Geometry: final body of the model. Coordinates: model frame, mm. A direction names the side the tool comes from. Coordinates: 2 decimals unless noted, no trailing zeros. Order: outer loops, then holes, each group sorted by start corner. A loop starts at its lowest first (then second) coordinate and runs counter-clockwise, first axis right, second up. Notation, with made-up numbers: (-8.5, -14) - (-0.5, -14) arc R20 cw to (-0.5, -8) - close; hole circle Ø7 at (-14, 89). An arc over 180 degrees is marked (long way). Use a Markdown table: item, result. Add a question column.
```python
from build123d import *

# Parameters (mm, degrees)
SKETCH1_R           = 34
SKETCH1_R_2         = 26.1
BOSS_EXTRUDE1_DEPTH = 5.5
SKETCH2_R           = 35.5
SKETCH2_R_2         = 25
BOSS_EXTRUDE2_DEPTH = 5.5
SKETCH3_R           = 25
SKETCH3_R_2         = 2.2
BOSS_EXTRUDE3_DEPTH = 5
CHAMFER1_SIZE       = 0.5
SKETCH5_R           = 2.5
SKETCH5_R_2         = 1.5
CUT_EXTRUDE1_DEPTH  = 17
SKETCH6_R           = 2.2
BOSS_EXTRUDE4_DEPTH = 20
SKETCH7_R           = 3.6
CUT_EXTRUDE2_DEPTH  = 4
SKETCH8_R           = 2.2
CUT_EXTRUDE3_DEPTH  = 8
SKETCH9_R           = 3.6
CUT_EXTRUDE4_DEPTH  = 4


with BuildPart() as part:
    # Sketch1 → Boss-Extrude1 (new body)
    with BuildSketch(Plane(origin=(0, 0, 0), x_dir=(1, 0, 0), z_dir=(0, 1, 0))):
        Circle(SKETCH1_R)
        Circle(SKETCH1_R_2, mode=Mode.SUBTRACT)
    extrude(amount=BOSS_EXTRUDE1_DEPTH)

    # Sketch2 → Boss-Extrude2 (add)
    with BuildSketch(Plane(origin=(0, 0, 0), x_dir=(-1, 0, 0), z_dir=(0, -1, 0))):
        Circle(SKETCH2_R)
        Circle(SKETCH2_R_2, mode=Mode.SUBTRACT)
    extrude(amount=BOSS_EXTRUDE2_DEPTH)

    # Sketch3 → Boss-Extrude3 (add)
    with BuildSketch(Plane.XZ.offset(5.5)):
        with BuildLine():
            Line((-55, -95), (-10, -95))
            ThreePointArc((-10, -95), (0, -85), (10, -95))
            Line((10, -95), (55, -95))
            Line((55, -95), (48.055, -75))
            Line((48.055, -75), (35.047098592, 5.652510971))
            ThreePointArc((35.047098592, 5.652510971), (0, 35.5), (-35.047098592, 5.652510971))
            Line((-35.047098592, 5.652510971), (-48.055, -75))
            Line((-48.055, -75), (-55, -95))
        make_face()
        Circle(SKETCH3_R, mode=Mode.SUBTRACT)
        with Locations((-25, -85)):
            Circle(SKETCH3_R_2, mode=Mode.SUBTRACT)
        with Locations((25, -85)):
            Circle(SKETCH3_R_2, mode=Mode.SUBTRACT)
    extrude(amount=BOSS_EXTRUDE3_DEPTH)

    # Chamfer1
    chamfer1_edges = [part.edges().sort_by_distance(p)[0] for p in [
        (-34, 0, 0),
        (-26.1, 5.5, 0),
    ]]
    chamfer(chamfer1_edges, length=CHAMFER1_SIZE)

    # Sketch5 → Cut-Extrude1 (cut, through all)
    with BuildSketch(Plane(origin=(0, 5.5, 0), x_dir=(1, 0, 0), z_dir=(0, 1, 0))):
        with Locations((21.213203436, 21.213203436)):
            Circle(SKETCH5_R)
        with Locations((0, 30)):
            Circle(SKETCH5_R_2)
        with Locations((30, 0)):
            Circle(SKETCH5_R_2)
        with Locations((0, -30)):
            Circle(SKETCH5_R_2)
        with Locations((-30, 0)):
            Circle(SKETCH5_R_2)
        with Locations((21.213203436, -21.213203436)):
            Circle(SKETCH5_R)
        with Locations((-21.213203436, -21.213203436)):
            Circle(SKETCH5_R)
        with Locations((-21.213203436, 21.213203436)):
            Circle(SKETCH5_R)
    extrude(amount=-CUT_EXTRUDE1_DEPTH, mode=Mode.SUBTRACT)

    # Sketch6 → Boss-Extrude4 (add)
    with BuildSketch(Plane(origin=(0, -5.5, 0), x_dir=(1, 0, 0), z_dir=(0, 1, 0))):
        with BuildLine():
            Line((52.222, 87), (55, 95))
            Line((55, 95), (10, 95))
            ThreePointArc((10, 95), (0, 85), (-10, 95))
            Line((-10, 95), (-55, 95))
            Line((-55, 95), (-52.222, 87))
            Line((-52.222, 87), (-38.747727085, 87))
            ThreePointArc((-38.747727085, 87), (-34.365946625, 85.693280212), (-31.415605973, 82.2))
            ThreePointArc((-31.415605973, 82.2), (-28.834057903, 79.143379814), (-25, 78))
            Line((-25, 78), (25, 78))
            ThreePointArc((25, 78), (28.834057903, 79.143379814), (31.415605973, 82.2))
            ThreePointArc((31.415605973, 82.2), (34.365946625, 85.693280212), (38.747727085, 87))
            Line((38.747727085, 87), (52.222, 87))
        make_face()
        with Locations((-25, 85)):
            Circle(SKETCH6_R, mode=Mode.SUBTRACT)
        with Locations((25, 85)):
            Circle(SKETCH6_R, mode=Mode.SUBTRACT)
    extrude(amount=BOSS_EXTRUDE4_DEPTH)

    # Sketch7 → Cut-Extrude2 (cut)
    with BuildSketch(Plane(origin=(0, 14.5, 0), x_dir=(1, 0, 0), z_dir=(0, 1, 0))):
        with Locations((25, 85)):
            Circle(SKETCH7_R)
        with Locations((-25, 85)):
            Circle(SKETCH7_R)
    extrude(amount=-CUT_EXTRUDE2_DEPTH, mode=Mode.SUBTRACT)

    # Sketch8 → Cut-Extrude3 (cut)
    with BuildSketch(Plane.XY.offset(-87)):
        with Locations((-45.484863542, 4.5)):
            Circle(SKETCH8_R)
        with Locations((45.484863542, 4.5)):
            Circle(SKETCH8_R)
    extrude(amount=-CUT_EXTRUDE3_DEPTH, mode=Mode.SUBTRACT)

    # Sketch9 → Cut-Extrude4 (cut)
    with BuildSketch(Plane.XY.offset(-87)):
        with Locations((-45.484863542, 4.5)):
            Circle(SKETCH9_R)
        with Locations((45.484863542, 4.5)):
            Circle(SKETCH9_R)
    extrude(amount=-CUT_EXTRUDE4_DEPTH, mode=Mode.SUBTRACT)


solid = part.part
```
1) Set-up query: faces 1 (the face through (34.312, 4.36, -85.658)), 2 (the face through (41.89, 4.66, -88.97)), 3 (the face through (-34.42, 4.36, -85.73)), 4 (the face through (24.53, 12.53, -88.57)). Return all of +Z, -Z, +X, -X, +Y, -Y with unobstructed straight access to the full face (end or side cutting, diameter ignored); none if empty.
2) Draft query along Y for faces 5 (the face through (20.671, -2.388, 23.654)), 6 (the face through (-1, -5.5, -50)), 7 (the face through (-42.05, 5.58, -88.97)). Return one class per face: pulls with the +Y half, pulls with the -Y half, needs draft (parallel to the pull), parting line crosses it, or undercut.
3) Section C-C (z = -52.5). Return loops of the section in (x, y), then the cut area to 3 significant figures.
4) Pin query (flat end, axial travel): pin 1 (8 mm diameter, centred on x = -27.5, y = -3.5, fed in from +Z); pin 2 (11 mm diameter, centred on x = 44.5, y = 2.5, fed in from +Z); pin 3 (1.5 mm diameter, centred on y = -1.5, z = 3.5, fed in from +X). Return the tip coordinate at first contact, or that it passes through.
5) Ray query, line 1 along Z through (x, y) = (0, -2.5); line 2 along X through (y, z) = (4.5, 0.5); line 3 along X through (y, z) = (-7.85, 0). Return the intervals inside material, ascending.
6) Section B-B (z = -80). Return loops of the section in (x, y).
7) Section A-A (x = 0). Give the number of separate pieces and of enclosed holes in the cut face, then the cut area to 3 significant figures.
Values follow:
| question | item | result |
|---|---|---|
| 1 | face 1 | +X, +Y |
| 1 | face 2 | +Z |
| 1 | face 3 | -X, +Y |
| 1 | face 4 | +Y |
| 2 | face 5 | needs draft |
| 2 | face 6 | pulls with the +Y half |
| 2 | face 7 | undercut |
| 3 | outline | (-44.43, -10.5) - (44.43, -10.5) - (44.43, -5.5) - (-44.43, -5.5) - close |
| 3 | area | 444 mm² |
| 4 | pin 1 | stops at z = 26.61 |
| 4 | pin 2 | stops at z = -87 |
| 4 | pin 3 | stops at x = 35.39 |
| 5 | line 1 | z = -85 to -78, -35.5 to -31.5, -28.5 to -25, 25 to 28.5, 31.5 to 35.5 |
| 5 | line 2 | x = -34 to -31.41, -28.59 to -26.1, 26.1 to 28.59, 31.41 to 34 |
| 5 | line 3 | x = -35.96 to -31.5, -28.5 to -25, 25 to 28.5, 31.5 to 35.96 |
| 6 | outline | (-49.79, -10.5) - (49.79, -10.5) - (49.79, -5.5) - (29.9, -5.5) - (29.9, 14.5) - (-29.9, 14.5) - (-29.9, -5.5) - (-49.79, -5.5) - close |
| 7 | separate pieces | 4 |
| 7 | enclosed holes | 0 |
| 7 | area | 599 mm² |
